Source: CAD feature listing. Evaluate the final solid. Frame: model axes, mm. A direction names the side the tool comes from. Round coordinates to 2 decimals unless told otherwise and drop trailing zeros. Write each loop counter-clockwise with the first axis right and the second up, starting at its lowest first coordinate (ties: lowest second). Pieces come first, ordered by that corner, then holes. Notation, with made-up numbers: M -32.5,35 L -13.5,35 A29 ccw -13.5,61 Z; hole C 38.5,62.25 d6. An arc over 180 degrees is marked long. Answer in a Markdown table with one row per item.
from build123d import *

# Parameters (mm, degrees)
SKETCH_1_W          = 4.5
SKETCH_1_H          = 28
EXTRUDE_1_DEPTH     = 3
SKETCH_4_W          = 50.1
SKETCH_4_H          = 22
EXTRUDE_2_DEPTH     = 3
SKETCH_5_W          = 4.5
SKETCH_5_H          = 28
EXTRUDE_3_DEPTH     = 3
SKETCH_6_R          = 1.25
CUT_EXTRUDE_2_DEPTH = 7
SKETCH_2_R          = 1.25
CUT_EXTRUDE_1_DEPTH = 4
SKETCH_7_R          = 5
SKETCH_7_R_2        = 1.25
CUT_EXTRUDE_3_DEPTH = 4
SKETCH_10_R         = 2.25
CUT_EXTRUDE_4_DEPTH = 3


with BuildPart() as part:
    # 스케치1 → 보스-돌출1 (new body)
    with BuildSketch(Plane.XY):
        with Locations((2.25, 14)):
            Rectangle(SKETCH_1_W, SKETCH_1_H)
    extrude(amount=EXTRUDE_1_DEPTH)

    # 스케치4 → 보스-돌출2 (add)
    with BuildSketch(Plane.XY.offset(3)):
        with Locations((25.05, 14)):
            Rectangle(SKETCH_4_W, SKETCH_4_H)
    extrude(amount=EXTRUDE_2_DEPTH)

    # 스케치5 → 보스-돌출3 (add)
    with BuildSketch(Plane(origin=(0, 0, 3), x_dir=(-1, 0, 0), z_dir=(0, 0, -1))):
        with Locations((-47.85, 14)):
            Rectangle(SKETCH_5_W, SKETCH_5_H)
    extrude(amount=EXTRUDE_3_DEPTH)

    # 스케치6 → 컷-돌출2 (cut, through all)
    with BuildSketch(Plane(origin=(0, 0, 0), x_dir=(-1, 0, 0), z_dir=(0, 0, -1))):
        with Locations((-47.85, 25)):
            Circle(SKETCH_6_R)
        with Locations((-47.85, 3)):
            Circle(SKETCH_6_R)
    extrude(amount=-CUT_EXTRUDE_2_DEPTH, mode=Mode.SUBTRACT)

    # 스케치2 → 컷-돌출1 (cut, through all)
    with BuildSketch(Plane.XY.offset(3)):
        with Locations((2.25, 25)):
            Circle(SKETCH_2_R)
        with Locations((2.25, 3)):
            Circle(SKETCH_2_R)
    extrude(amount=-CUT_EXTRUDE_1_DEPTH, mode=Mode.SUBTRACT)

    # 스케치7 → 컷-돌출3 (cut, through all)
    with BuildSketch(Plane(origin=(0, 0, 3), x_dir=(-1, 0, 0), z_dir=(0, 0, -1))):
        with Locations((-25.05, 14)):
            Circle(SKETCH_7_R)
        with Locations((-36.05, 20)):
            Circle(SKETCH_7_R_2)
        with Locations((-14.05, 20)):
            Circle(SKETCH_7_R_2)
        with Locations((-36.05, 8)):
            Circle(SKETCH_7_R_2)
        with Locations((-14.05, 8)):
            Circle(SKETCH_7_R_2)
    extrude(amount=-CUT_EXTRUDE_3_DEPTH, mode=Mode.SUBTRACT)

    # 스케치10 → 컷-돌출4 (cut)
    with BuildSketch(Plane.XY.offset(6)):
        with Locations((2.25, 25)):
            Circle(SKETCH_10_R)
        with Locations((2.25, 3)):
            Circle(SKETCH_10_R)
        with Locations((47.85, 25)):
            Circle(SKETCH_10_R)
        with Locations((47.85, 3)):
            Circle(SKETCH_10_R)
    extrude(amount=-CUT_EXTRUDE_4_DEPTH, mode=Mode.SUBTRACT)


solid = part.part
Q1. Section C-C (y = 17.25). Return loops of the section in (x, z).
Solutions:
| item | result |
|---|---|
| outline | M 0,0 L 4.5,0 L 4.5,3 L 21.25,3 L 21.25,6 L 0,6 Z; M 28.85,3 L 45.6,3 L 45.6,0 L 50.1,0 L 50.1,6 L 28.85,6 Z |
Q2. Material intervals for probe 1 along Y at (x, z) = (47.85, 1.95); probe 2 along Y at (x, z) = (36.05, 3.75); probe 3 along X at (y, z) = (26.75, 1.1), sorted ascending.
Solutions:
| item | result |
|---|---|
| probe 1 | y = 0 to 1.75, 4.25 to 23.75, 26.25 to 28 |
| probe 2 | y = 3 to 6.75, 9.25 to 18.75, 21.25 to 25 |
| probe 3 | x = 0 to 4.5, 45.6 to 50.1 |
Q3. Section D-D (x = 25.05). Return loops of the section in (y, z), and give its area (3 significant figures).
Solutions:
| item | result |
|---|---|
| outline | M 3,3 L 9,3 L 9,6 L 3,6 Z; M 19,3 L 25,3 L 25,6 L 19,6 Z |
| area | 36.0 mm2 |
Q4. Section A-A (z = 1.7). Return loops of the section in (x, y).
Solutions:
| item | result |
|---|---|
| outline | M 0,0 L 4.5,0 L 4.5,28 L 0,28 Z; M 45.6,0 L 50.1,0 L 50.1,28 L 45.6,28 Z; hole C 2.25,3 d2.5; hole C 2.25,25 d2.5; hole C 47.85,3 d2.5; hole C 47.85,25 d2.5 |
Q5. Contact query for flat-ended pins moving along their axis: pin 1 Ø2 at (x, y) = (47, 4) entering from +Z; pin 2 Ø3.5 at (x, z) = (35.5, 5) entering from -Y; pin 3 Ø4 at (x, y) = (47.85, 3) entering from +Z; pin 4 Ø6.5 at (x, y) = (21.5, 11) entering from -Z. Output: stop coordinate, or through.
Solutions:
| item | result |
|---|---|
| pin 1 | stops at z = 6 |
| pin 2 | stops at y = 3 |
| pin 3 | stops at z = 3 |
| pin 4 | stops at z = 3 |
Q6. Pull-direction query (Y, two-part tool) for faces 1 (the cylindrical face through (14.32, 18.78, 4.48)), 2 (the flat face through (2, 0, 1)), 3 (the flat face through (48, 28, 2)); classes: pulls with the +Y half, pulls with the -Y half, needs draft (parallel to the pull), parting line crosses it, or undercut.
Solutions:
| item | result |
|---|---|
| face 1 | undercut |
| face 2 | pulls with the -Y half |
| face 3 | pulls with the +Y half |
Q7. Access query for faces 4 (the cylindrical face through (47.9, 5.25, 4.52)), 5 (the flat face through (4.5, 14, 1)), 6 (the flat face through (48, 27, 3)), 7 (the flat face through (19, 14, 6)). Directions: +Z, -Z, +X, -X, +Y, -Y. A direction counts if a zero-diameter tool reaches every point of the face in a straight line with its end or side. Return the directions, or none.
Solutions:
| item | result |
|---|---|
| face 4 | +Z, -Y |
| face 5 | -Z, +Y, -Y |
| face 6 | +Z, +Y |
| face 7 | +Z, +X, -X, +Y, -Y |
Q8. Section B-B (x = 14.05). Return loops of the section in (y, z), and give its area (3 significant figures).
Solutions:
| item | result |
|---|---|
| outline | M 3,3 L 6.75,3 L 6.75,6 L 3,6 Z; M 9.25,3 L 18.75,3 L 18.75,6 L 9.25,6 Z; M 21.25,3 L 25,3 L 25,6 L 21.25,6 Z |
| area | 51.0 mm2 |
